Autodesk Inventor part; units mm, degrees
ref_plane "Belt Plane" through (0, 53.5, 8) normal (0, 0, 1) x (1, 0, 0)
ref_plane "YZ Plane" through (0, 0, 0) normal (1, 0, 0) x (0, 1, 0)
ref_plane "XZ Plane" through (0, 0, 0) normal (0, 1, 0) x (-1, 0, 0)
sketch "Main Sketch" plane through (0, 0, 0) normal (1, 0, 0) x (0, 1, 0)
  line L0 (0, 28) -> (64.5, 28)
  line L1 (64.5, 28) -> (64.5, 12.9387)
  line L2 (64.5, 12.9387) -> (53.5, 9.1511)
  line L3 (53.5, 9.1511) -> (53.5, 6.8489)
  line L4 (53.5, 6.8489) -> (64.5, 3.0613)
  line L5 (64.5, 3.0613) -> (64.5, 0)
  line L6 (64.5, 0) -> (0, 0)
  line L7 (62.5, 12.25) -> (62.5, 3.75) construction
  line L8 (53.5, 8) -> (62.5, 8) construction
  line L9 (64.5, 12.9387) -> (64.5, 3.0613)
  line L10 (0, -4) -> (0, 24)
  line L11 (0, 0) -> (0, 28)
  dimension "d0" = 8.5
  dimension "d1" = 38
  dimension "d2" = 2
  dimension "d6" = 28
  dimension "d21" = 125
  dimension "d25" = 11
  dimension "d27" = 8
ref_plane "Belt Plane" through (0, 53.5, 8) normal (0, 0, 1) x (1, 0, 0)
revolve "Body" add sketch "Main Sketch" angle 360 about axis through (0, 0, -10) along (0, 0, 1)
revolve "Groove" cut sketch "Main Sketch" angle 360 about axis through (0, 0, -10) along (0, 0, 1) contours L9 L4 L3 L2
fillet "Fillet External" [suppressed]
fillet "Fillet Internal" [suppressed]
pattern_linear "Groove Pattern" count 2 spacing 12 along (0, 0, 1) of "Groove"
equation "\"d0\" = da_Bw"
equation "\"d1\" = da_Alfa"
equation "\"d2\" = da_c"
equation "\"d21\" = da_Dw"
equation "\"d25\" = da_Hd"
equation "\"d27\" = da_Se"
equation "\"da_r1\" = 0"
equation "\"da_r2\" = 0"
equation "\"d18\" = da_Sg"
equation "\"d5\" = da_Se"
equation "\"da_Bw\" = 8.5"
equation "\"da_Alfa\" = 38deg"
equation "\"da_c\" = 2"
equation "\"da_Dw\" = 125"
equation "\"da_Hd\" = 11"
equation "\"da_Se\" = 8"
equation "\"da_Sg\" = 12"
properties part number "Grooved Pulley1" material "Steel"
Work out the finished part from the listing and answer in its coordinate system (mm). A direction names the side the tool comes from. Coordinates: 2 decimals unless noted, no trailing zeros. Loops run counter-clockwise (first coordinate to the right, second up) from the corner with the lowest first, then second, coordinate; pieces in that order, holes last. Notation, with made-up numbers: M 71.25,49.25 L 82.25,49.25 A22 cw 82.25,78.25 Z; hole C 38,18.5 d2. An arc over 180 degrees is marked long. Answer in a Markdown table with one row per item. Add a question column.
1. A tool of negligible diameter and unlimited length cuts with its end or side. For faces 5 (the conical face through (52.9, -11.75, 21.39)), 6 (the cylindrical face through (19.374, 61.522, 13.985)), from which of +Z, -Z, +X, -X, +Y, -Y can it reach the whole face along a straight path? Write none if from no direction.
2. Find section A-A, the plane y = 0. Write down the section's boundary in (x, z).
3. Consider L1, parallel to Z at x = 59, y = 18.5; L2, parallel to Z at x = -31, y = 44; L3, parallel to Y at x = -40, z = 19.5. Determine where each line is inside the solid, lowest interval first.
4. Find section C-C, the plane z = 22.75. Write down the section's boundary in (x, y).
5. Flat-ended cylindrical pins translate along their axes: P1, Ø6, axis at y = -39.5, z = 25, coming from the +X side; P2, Ø12, axis at y = -4, z = 8, coming from the +X side; P3, Ø1.5, axis at x = -17.5, z = 15, coming from the -Y side. Find the tip coordinate at first contact, or state that the pin passes through.
6. The mould has two halves that part along Z. Classify faces 1 (the flat face through (-1, -1, 28)), 2 (the flat face through (-1, -1, 0)), 3 (the cylindrical face through (19.374, 61.522, 1.509)), 4 (the cylindrical face through (-52.228, -11.598, 19.984)): pulls with the +Z half, pulls with the -Z half, needs draft (parallel to the pull), parting line crosses it, or undercut.
Reported:
| question | item | result |
|---|---|---|
| 1 | face 5 | none |
| 1 | face 6 | +Z, -Z |
| 2 | outline | M -64.5,0 L 64.5,0 L 64.5,3.06 L 53.5,6.85 L 53.5,9.15 L 64.5,12.94 L 64.5,15.06 L 53.5,18.85 L 53.5,21.15 L 64.5,24.94 L 64.5,28 L -64.5,28 L -64.5,24.94 L -53.5,21.15 L -53.5,18.85 L -64.5,15.06 L -64.5,12.94 L -53.5,9.15 L -53.5,6.85 L -64.5,3.06 Z |
| 3 | L1 | z = 0 to 3.98, 12.02 to 15.98, 24.02 to 28 |
| 3 | L2 | z = 0 to 6.74, 9.26 to 18.74, 21.26 to 28 |
| 3 | L3 | y = -35.53 to 35.53 |
| 4 | outline | C 0,0 d116.29 |
| 5 | P1 | stops at x = 53.18 |
| 5 | P2 | stops at x = 64.5 |
| 5 | P3 | stops at y = -62.29 |
| 6 | face 1 | pulls with the +Z half |
| 6 | face 2 | pulls with the -Z half |
| 6 | face 3 | needs draft |
| 6 | face 4 | undercut |
